The model under review builds one solid part; all positions refer to its coordinate system, in mm. Coordinates: 2 decimals unless noted, no trailing zeros. Order: outer loops, then holes, each group sorted by start corner. A loop starts at its lowest first (then second) coordinate and runs counter-clockwise, first axis right, second up. Notation, with made-up numbers: M 71,-35.5 L 130,-35.5 A16 cw 130,-6.5 Z; hole C -1.75,13 d7. An arc over 180 degrees is marked long. Answer in a Markdown table with one row per item.
from build123d import *

# Parameters (mm, degrees)
SKIZZE3_W                            = 23
SKIZZE3_H                            = 5
AUFSATZ_LINEAR_AUSTRAGEN1_DEPTH      = 15
AUFSATZ_LINEAR_AUSTRAGEN1_DEPTH_BACK = 15
SKIZZE5_R                            = 3
SCHNITT_LINEAR_AUSTRAGEN1_DEPTH      = 16


with BuildPart() as part:
    # Skizze3 → Aufsatz-Linear austragen1 (new body, two sides)
    with BuildSketch(Plane.XY) as aufsatz_linear_austragen1_sk:
        with Locations((-53.5, -13.5)):
            Rectangle(SKIZZE3_W, SKIZZE3_H)
    extrude(amount=AUFSATZ_LINEAR_AUSTRAGEN1_DEPTH)
    extrude(aufsatz_linear_austragen1_sk.sketch, amount=-AUFSATZ_LINEAR_AUSTRAGEN1_DEPTH_BACK)

    # Skizze5 → Schnitt-Linear austragen1 (cut)
    with BuildSketch(Plane(origin=(0, 0, 0), x_dir=(1, 0, 0), z_dir=(0, 1, 0))):
        with Locations((-53, 7.5)):
            Circle(SKIZZE5_R)
        with Locations((-53, -7.5)):
            Circle(SKIZZE5_R)
    extrude(amount=-SCHNITT_LINEAR_AUSTRAGEN1_DEPTH, mode=Mode.SUBTRACT)


solid = part.part
(1) Take a section at B-B (z = -7.5). Write out the cut boundary in (x, y), then the cut area to 3 significant figures.
Report:
| item | result |
|---|---|
| outline | M -65,-16 L -56,-16 L -56,-11 L -65,-11 Z; M -50,-16 L -42,-16 L -42,-11 L -50,-11 Z |
| area | 85.0 mm^2 |
(2) To check wall thickness, follow line 1 (Z direction, x = -53, y = -14.2); line 2 (X direction, y = -12.05, z = -7.5); line 3 (X direction, y = -11.3, z = -9.75). State the ranges of each line that lie inside material, in increasing order. Write a range as [from, to].
Report:
| item | result |
|---|---|
| line 1 | [-15, -10.5], [-4.5, 4.5], [10.5, 15] |
| line 2 | [-65, -56], [-50, -42] |
| line 3 | [-65, -54.98], [-51.02, -42] |
(3) Take a section at A-A (x = -53). Write out the cut boundary in (y, z).
Report:
| item | result |
|---|---|
| outline | M -16,-15 L -11,-15 L -11,-10.5 L -16,-10.5 Z; M -16,-4.5 L -11,-4.5 L -11,4.5 L -16,4.5 Z; M -16,10.5 L -11,10.5 L -11,15 L -16,15 Z |
(4) The part is to be moulded in two halves that separate along X. For faces 1 (the flat face through (-54, -13, -15)), 2 (the flat face through (-42, -14, 0)), 3 (the cylindrical face through (-56, -13.5, 7.4)), say which applies: +X half, -X half, draft (parallel to the pull), parting line (faces both ways), or undercut.
Report:
| item | result |
|---|---|
| face 1 | draft |
| face 2 | +X half |
| face 3 | undercut |
(5) Take a section at C-C (y = -14). Write out the cut boundary in (x, z), then the cut area to 3 significant figures.
Report:
| item | result |
|---|---|
| outline | M -65,-15 L -42,-15 L -42,15 L -65,15 Z; hole C -53,-7.5 d6; hole C -53,7.5 d6 |
| area | 633 mm^2 |
